```python
from build123d import *

# Parameters (mm, degrees)
MODEL_W                     = 160
MODEL_H                     = 80
MODEL_R                     = 2.55
MODEL_R_2                   = 1.8
MODEL_R_3                   = 2.5
MODEL_R_4                   = 3.5
MODEL_R_5                   = 2.015564
DODANIE_WYCI_GNI_CIE1_DEPTH = 1.5
MODEL_3_R                   = 2.015564
MODEL_3_R_2                 = 3.5
DODANIE_WYCI_GNI_CIE2_DEPTH = 6
MODEL_4_R                   = 2.5
DODANIE_WYCI_GNI_CIE3_DEPTH = 19
ZAOKR_GLENIE1_R             = 2
MODEL_5_W                   = 98
MODEL_5_H                   = 60
DODANIE_WYCI_GNI_CIE4_DEPTH = 18
MODEL_6_W                   = 97
MODEL_6_H                   = 39.5
DODANIE_WYCI_GNI_CIE5_DEPTH = 28
SZKIC2_W                    = 76
SZKIC2_H                    = 25
WYTNIJ_WYCI_GNI_CIE1_DEPTH  = 1
ZAOKR_GLENIE2_R             = 0.5
DODANIE_WYCI_GNI_CIE6_START = 3
SZKIC3_W                    = 20
SZKIC3_H                    = 33.5
DODANIE_WYCI_GNI_CIE6_DEPTH = 1.5


with BuildPart() as part:
    # Model → Dodanie-wyci_gni_cie1 (new body)
    with BuildSketch(Plane.XY):
        with Locations((80, 40)):
            Rectangle(MODEL_W, MODEL_H)
        with Locations((14.5, 64.5)):
            Circle(MODEL_R, mode=Mode.SUBTRACT)
        with Locations((4, 4)):
            Circle(MODEL_R_2, mode=Mode.SUBTRACT)
        with Locations((154.00374, 64.012896)):
            Circle(MODEL_R_3, mode=Mode.SUBTRACT)
        with Locations((14.5, 9.5)):
            Circle(MODEL_R, mode=Mode.SUBTRACT)
        with Locations((107.5, 9.5)):
            Circle(MODEL_R, mode=Mode.SUBTRACT)
        with Locations((107.5, 64.5)):
            Circle(MODEL_R, mode=Mode.SUBTRACT)
        with Locations((156, 76)):
            Circle(MODEL_R_2, mode=Mode.SUBTRACT)
        with Locations((156, 4)):
            Circle(MODEL_R_2, mode=Mode.SUBTRACT)
        with Locations((137.7008, 12)):
            Circle(MODEL_R_4, mode=Mode.SUBTRACT)
        with Locations((137.989674, 33.022353)):
            Circle(MODEL_R_5, mode=Mode.SUBTRACT)
        with Locations((4, 76)):
            Circle(MODEL_R_2, mode=Mode.SUBTRACT)
        with Locations((123.499421, 45.511083)):
            Circle(MODEL_R_5, mode=Mode.SUBTRACT)
        with Locations((152.465613, 45.526919)):
            Circle(MODEL_R_5, mode=Mode.SUBTRACT)
        with Locations((138, 58)):
            Circle(MODEL_R_5, mode=Mode.SUBTRACT)
        with Locations((121.957824, 63.96421)):
            Circle(MODEL_R_3, mode=Mode.SUBTRACT)
        Polygon((109.5, 56.75), (109.5, 17.25), (12.5, 17.25), (12.5, 56.75), (70.19, 56.75), (70.19, 57.27), (79.715, 57.27), (80.235, 56.75), align=None, mode=Mode.SUBTRACT)
    extrude(amount=DODANIE_WYCI_GNI_CIE1_DEPTH)

    # Model_3 → Dodanie-wyci_gni_cie2 (add)
    with BuildSketch(Plane.XY):
        with Locations((138, 58)):
            Circle(MODEL_3_R)
        with Locations((123.499421, 45.511083)):
            Circle(MODEL_3_R)
        with Locations((152.465613, 45.526919)):
            Circle(MODEL_3_R)
        with Locations((137.7008, 12)):
            Circle(MODEL_3_R_2)
        with Locations((137.989674, 33.022353)):
            Circle(MODEL_3_R)
    extrude(amount=DODANIE_WYCI_GNI_CIE2_DEPTH)

    # Model_4 → Dodanie-wyci_gni_cie3 (add)
    with BuildSketch(Plane.XY):
        with Locations((121.957824, 63.96421)):
            Circle(MODEL_4_R)
        with Locations((154.00374, 64.012896)):
            Circle(MODEL_4_R)
    extrude(amount=DODANIE_WYCI_GNI_CIE3_DEPTH)

    # Zaokr_glenie1
    zaokr_glenie1_edges = [part.edges().sort_by_distance(p)[0] for p in [
        (119.457824, 63.96421, 19),
        (151.50374, 64.012896, 19),
    ]]
    fillet(zaokr_glenie1_edges, radius=ZAOKR_GLENIE1_R)

    # Model_5 → Dodanie-wyci_gni_cie4 (add)
    with BuildSketch(Plane.XY):
        with Locations((61, 37)):
            Rectangle(MODEL_5_W, MODEL_5_H)
    extrude(amount=DODANIE_WYCI_GNI_CIE4_DEPTH)

    # Model_6 → Dodanie-wyci_gni_cie5 (add)
    with BuildSketch(Plane.XY):
        with Locations((61, 37)):
            Rectangle(MODEL_6_W, MODEL_6_H)
    extrude(amount=DODANIE_WYCI_GNI_CIE5_DEPTH)

    # Szkic2 → Wytnij-wyci_gni_cie1 (cut)
    with BuildSketch(Plane.XY.offset(28)):
        with Locations((61, 37)):
            Rectangle(SZKIC2_W, SZKIC2_H)
    extrude(amount=-WYTNIJ_WYCI_GNI_CIE1_DEPTH, mode=Mode.SUBTRACT)

    # Zaokr_glenie2
    zaokr_glenie2_edges = [part.edges().sort_by_distance(p)[0] for p in [
        (12.5, 37, 28),
        (61, 17.25, 28),
        (109.5, 37, 28),
        (61, 56.75, 28),
    ]]
    fillet(zaokr_glenie2_edges, radius=ZAOKR_GLENIE2_R)

    # Szkic3 → Dodanie-wyci_gni_cie6 (add)
    with BuildSketch(Plane.XY.offset(1.5).offset(DODANIE_WYCI_GNI_CIE6_START)):
        with Locations((75.27, 67.75)):
            Rectangle(SZKIC3_W, SZKIC3_H)
    extrude(amount=DODANIE_WYCI_GNI_CIE6_DEPTH)


solid = part.part
```
Source: CAD feature listing. Evaluate the final solid. Frame: model axes, mm. A direction names the side the tool comes from. Give positions to 0.01 mm unless a question says otherwise; leave off trailing zeros. Order: outer loops, then holes, each group sorted by start corner. A loop starts at its lowest first (then second) coordinate and runs counter-clockwise, first axis right, second up.
(1) Contact query for flat-ended pins moving along their axis: P1, Ø9, axis at x = 79.5, z = 8.5, coming from the -Y side; P2, Ø8, axis at x = 94, y = 61.5, coming from the +Z side; P3, Ø0.5, axis at y = 35, z = 27.5, coming from the +X side; P4, Ø6, axis at y = 72.5, z = 4, coming from the +X side. Output: stop coordinate, or through.
(2) Section query A-A (y = 76). Return the cut outline in (x, z).
(3) Section query B-B (x = 26.5). Return the cut outline in (y, z).
(4) Pull-direction query (Y, two-part tool) for faces 4 (the face through (109.5, 37, 23)), 5 (the face through (60, 17.25, 23)), 6 (the face through (135.976, 33.111, 3.718)); classes: +Y half, -Y half, draft (parallel to the pull), parting line (faces both ways), or undercut.
(5) Access query for faces 1 (the face through (151.506, 64.123, 9.142)), 2 (the face through (152, 46, 6)), 3 (the face through (138, 58, 6)). Directions: +Z, -Z, +X, -X, +Y, -Y. A direction counts if a zero-diameter tool reaches every point of the face in a straight line with its end or side. Return the directions, or none.
(6) Material intervals for line 1 along Y through (x, z) = (156, 0.9); line 2 along X through (y, z) = (76, 1.2); line 3 along Y through (x, z) = (55.5, 25.25), sorted ascending.
(7) Section query D-D (y = 4). Return the cut outline in (x, z), plus the area to 3 significant figures.
(8) Section query C-C (y = 41.5). Return the cut outline in (x, z).
Outcome:
1. P1: stops at y = 7
1. P2: stops at z = 18
1. P3: stops at x = 109.5
1. P4: stops at x = 160
2. outline: (0, 0) - (2.2, 0) - (2.2, 1.5) - (0, 1.5) - close; (5.8, 0) - (154.2, 0) - (154.2, 1.5) - (5.8, 1.5) - close; (65.27, 4.5) - (85.27, 4.5) - (85.27, 6) - (65.27, 6) - close; (157.8, 0) - (160, 0) - (160, 1.5) - (157.8, 1.5) - close
3. outline: (0, 0) - (80, 0) - (80, 1.5) - (67, 1.5) - (67, 18) - (56.75, 18) - (56.75, 27.5) arc R0.5 ccw to (56.25, 28) - (49.5, 28) - (49.5, 27) - (24.5, 27) - (24.5, 28) - (17.75, 28) arc R0.5 ccw to (17.25, 27.5) - (17.25, 18) - (7, 18) - (7, 1.5) - (0, 1.5) - close
4. face 4: draft
4. face 5: -Y half
4. face 6: undercut
5. face 1: +Z
5. face 2: +Z, +X, -Y
5. face 3: +Z, +X, +Y, -Y
6. line 1: y = 0 to 2.2, 5.8 to 74.2, 77.8 to 80
6. line 2: x = 0 to 2.2, 5.8 to 154.2, 157.8 to 160
6. line 3: y = 17.25 to 56.75
7. outline: (0, 0) - (2.2, 0) - (2.2, 1.5) - (0, 1.5) - close; (5.8, 0) - (154.2, 0) - (154.2, 1.5) - (5.8, 1.5) - close; (157.8, 0) - (160, 0) - (160, 1.5) - (157.8, 1.5) - close
7. area: 229 mm2
8. outline: (0, 0) - (160, 0) - (160, 1.5) - (110, 1.5) - (110, 18) - (109.5, 18) - (109.5, 27.5) arc R0.5 ccw to (109, 28) - (99, 28) - (99, 27) - (23, 27) - (23, 28) - (13, 28) arc R0.5 ccw to (12.5, 27.5) - (12.5, 18) - (12, 18) - (12, 1.5) - (0, 1.5) - close
